Check sheet for the modelled part. Datum: model origin and axes. Units: mm. Give positions to 0.01 mm unless a question says otherwise; leave off trailing zeros. Write each loop counter-clockwise with the first axis right and the second up, starting at its lowest first coordinate (ties: lowest second). Pieces come first, ordered by that corner, then holes. Notation, with made-up numbers: M 73.25,65.5 L 118.25,65.5 A9 cw 118.25,76.5 Z; hole C 8.25,65.25 d2. An arc over 180 degrees is marked long. Write each question's results on one line, items separated by ' | '. Start each with the question number.
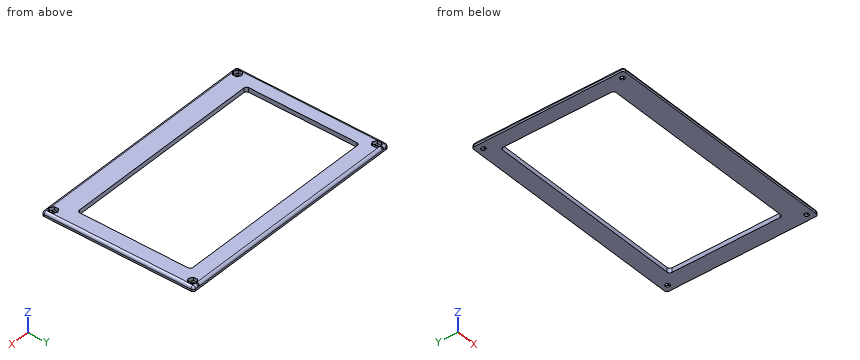
Autodesk Inventor part; units mm, degrees
ref_plane "YZ Plane" through (0, 0, 0) normal (1, 0, 0) x (0, 1, 0)
ref_plane "XZ Plane" through (0, 0, 0) normal (0, 1, 0) x (-1, 0, 0)
ref_plane "XY Plane" through (0, 0, 0) normal (0, 0, 1) x (1, 0, 0)
sketch "Sketch1" plane through (0, 0, 0) normal (0, 0, 1) x (1, 0, 0)
  circle A0 centre (86.5, 54) radius 1.75
  circle A1 centre (-86.5, 54) radius 1.75
  circle A2 centre (86.5, -54) radius 1.75
  circle A3 centre (-86.5, -54) radius 1.75
  line L0 (91.5, 59) -> (-91.5, 59)
  line L1 (-91.5, 59) -> (-91.5, -59)
  line L2 (-91.5, -59) -> (91.5, -59)
  line L3 (91.5, -59) -> (91.5, 59)
  line L4 (78.5, -42) -> (-80, -42)
  circle A4 centre (86.5, 54) radius 1.75
  circle A5 centre (-86.5, 54) radius 1.75
  circle A6 centre (86.5, -54) radius 1.75
  circle A7 centre (-86.5, -54) radius 1.75
  line L5 (91.5, 59) -> (-91.5, 59)
  line L6 (-91.5, 59) -> (-91.5, -59)
  line L7 (-91.5, -59) -> (91.5, -59)
  line L8 (91.5, -59) -> (91.5, 59)
  line L9 (78.5, 46) -> (78.5, -42)
  line L10 (-80, -42) -> (-80, 46)
  line L11 (-128.1, 0) -> (128.1, 0)
  line L12 (0, -82.95) -> (0, 84.7)
  line L13 (-80, 46) -> (78.5, 46)
  line L14 (84.25, 60.75) -> (84.25, 59)
  line L15 (78.5, 46) -> (78.5, -42)
  line L16 (-80, -42) -> (-80, 46)
  line L17 (-84.25, 59) -> (-84.25, 60.75)
  point P0 (0, 0)
  point P1 (0, 0)
  point P2 (0, 0)
  dimension "d0" = 183
  dimension "d1" = 118
  dimension "d2" = 3.5
  dimension "d3" = 17
  dimension "d4" = 13
  dimension "d5" = 13
  dimension "d6" = 11.5
extrude "Extrusion1" add sketch "Sketch1" along normal blind 3.5 contours L3 L11 L9 L13 L12 L0 | L3 L2 L12 L4 L9 L11 | L12 L13 L10 L11 L1 L0 | L2 L1 L11 L10 L4 L12
sketch "Sketch2" plane through (0, 0, 3.5) normal (0, 0, 1) x (1, 0, 0)
  line L0 (-80, 46) -> (78.5, 46)
  line L1 (78.5, 46) -> (78.5, -42)
  line L2 (78.5, -42) -> (-80, -42)
  line L3 (-80, -42) -> (-80, 46)
  circle A0 centre (-86.5, -54) radius 1.75
  circle A1 centre (86.5, -54) radius 1.75
  circle A2 centre (-86.5, 54) radius 1.75
  circle A3 centre (86.5, 54) radius 1.75
  line L4 (91.5, 59) -> (-91.5, 59)
  line L5 (-91.5, 59) -> (-91.5, -59)
  line L6 (-91.5, -59) -> (91.5, -59)
  line L7 (91.5, -59) -> (91.5, 59)
  circle A4 centre (86.5, 54) radius 1.75
  circle A5 centre (86.5, 54) radius 1.75
  line L8 (83.5772, 55.6875) -> (86.5, 57.375)
  line L9 (86.5, 57.375) -> (89.4228, 55.6875)
  line L10 (89.4228, 55.6875) -> (89.4228, 52.3125)
  line L11 (89.4228, 52.3125) -> (86.5, 50.625)
  line L12 (86.5, 50.625) -> (83.5772, 52.3125)
  line L13 (83.5772, 52.3125) -> (83.5772, 55.6875)
  circle A6 centre (86.5, 54) radius 3.375 construction
  line L14 (-89.4228, 52.3125) -> (-89.4228, 55.6875)
  line L15 (-89.4228, 55.6875) -> (-86.5, 57.375)
  line L16 (-86.5, 57.375) -> (-83.5772, 55.6875)
  line L17 (-83.5772, 55.6875) -> (-83.5772, 52.3125)
  line L18 (-83.5772, 52.3125) -> (-86.5, 50.625)
  line L19 (-86.5, 50.625) -> (-89.4228, 52.3125)
  line L20 (-86.5, -57.375) -> (-89.4228, -55.6875)
  line L21 (-89.4228, -55.6875) -> (-89.4228, -52.3125)
  line L22 (-89.4228, -52.3125) -> (-86.5, -50.625)
  line L23 (-86.5, -50.625) -> (-83.5772, -52.3125)
  line L24 (-83.5772, -52.3125) -> (-83.5772, -55.6875)
  line L25 (-83.5772, -55.6875) -> (-86.5, -57.375)
  line L26 (83.5772, -55.6875) -> (83.5772, -52.3125)
  line L27 (83.5772, -52.3125) -> (86.5, -50.625)
  line L28 (86.5, -50.625) -> (89.4228, -52.3125)
  line L29 (89.4228, -52.3125) -> (89.4228, -55.6875)
  line L30 (89.4228, -55.6875) -> (86.5, -57.375)
  line L31 (86.5, -57.375) -> (83.5772, -55.6875)
  point P0 (0, 0)
  point P1 (89.4228, 54)
  point P2 (-83.5772, 54)
  point P3 (-83.5772, -54)
  point P4 (89.4228, -54)
  dimension "d9" = 6.75
  dimension "d12" = 173
  dimension "d19" = 108
extrude "Extrusion3" cut sketch "Sketch2" against normal blind 2.5 contours L8 L9 L10 L11 L12 L13 | L14 L15 L16 L17 L18 L19 | L20 L21 L22 L23 L24 L25 | L26 L27 L28 L29 L30 L31
fillet "Fillet1" radius 2 12 edges at (-91.5, -59, 1.75) (91.5, -59, 1.75) (-91.5, 59, 1.75) (91.5, 59, 1.75) (91.5, 0, 3.5) (0, 59, 3.5) (-91.5, 0, 3.5) (0, -59, 3.5) (-80, 46, 1.75) (78.5, 46, 1.75) (78.5, -42, 1.75) (-80, -42, 1.75)
properties part number "tapa"
Q1. Section check A-A on y = 17. Record the boundary of the cut face in (x, z), plus the area to 3 significant figures.
Q2. Depth check by flat-ended pin: pin 1 Ø5.5 at (x, y) = (-86.5, -54) entering from +Z; pin 2 Ø1.2 at (y, z) = (53.5, 2.5) entering from -X; pin 3 Ø1.5 at (x, z) = (38.5, 2.5) entering from +Y. Enter the tip coordinate at first touch or a pass-through.
Q3. Scan lines: L1, parallel to Y at x = 86.5, z = 0.35; L2, parallel to X at y = 51, z = 1.9; L3, parallel to Y at x = -62.5, z = 0.35. Record each from-to range of solid material in increasing order.
Q4. Section check C-C on z = 2.85. State how many separate pieces and enclosed holes the cut face has, plus the area to 3 significant figures.
Q5. Section check B-B on x = -71.5. Record the boundary of the cut face in (y, z), plus the area to 3 significant figures.
Check result:
1) outline: M -91.5,0 L -80,0 L -80,3.5 L -89.5,3.5 A2 ccw -91.5,1.5 Z; M 78.5,0 L 91.5,0 L 91.5,1.5 A2 ccw 89.5,3.5 L 78.5,3.5 Z | area: 84.0 mm^2
2) pin 1: z = 1 | pin 2: x = -91.46 | pin 3: y = 58.98
3) L1: -59 to -55.75, -52.25 to 52.25, 55.75 to 59 | L2: -91.46 to -87.15, -85.85 to 85.85, 87.15 to 91.46 | L3: -59 to -42, 46 to 59
4) separate pieces: 1 | enclosed holes: 5 | area: 7,210 mm^2
5) outline: M -59,0 L -42,0 L -42,3.5 L -57,3.5 A2 ccw -59,1.5 Z; M 46,0 L 59,0 L 59,1.5 A2 ccw 57,3.5 L 46,3.5 Z | area: 103 mm^2
